```python
from build123d import *

# Parameters (mm, degrees)
SKETCH1_R           = 127.525
SKETCH1_R_2         = 124.525
BOSS_EXTRUDE1_DEPTH = 3
SKETCH2_R           = 1.5
BOSS_EXTRUDE2_DEPTH = 3
BOSS_EXTRUDE3_DEPTH = 3
FILLET1_R           = 5


with BuildPart() as part:
    # Sketch1 → Boss-Extrude1 (new body)
    with BuildSketch(Plane.XY):
        Circle(SKETCH1_R)
        Circle(SKETCH1_R_2, mode=Mode.SUBTRACT)
    extrude(amount=BOSS_EXTRUDE1_DEPTH)

    # Sketch2 → Boss-Extrude2 (add)
    with BuildSketch(Plane.XY.offset(3)):
        with BuildLine():
            Line((-6.110237311, 124.375), (-5, 119.525))
            ThreePointArc((-5, 119.525), (0, 114.525), (5, 119.525))
            Line((5, 119.525), (6.110237311, 124.375))
            ThreePointArc((6.110237311, 124.375), (0, 124.525), (-6.110237311, 124.375))
        make_face()
        with Locations((0, 119.525)):
            Circle(SKETCH2_R, mode=Mode.SUBTRACT)
        with BuildLine():
            Line((-119.525, 5), (-124.375, 6.110237311))
            ThreePointArc((-124.375, 6.110237311), (-124.525, 0), (-124.375, -6.110237311))
            Line((-124.375, -6.110237311), (-119.525, -5))
            ThreePointArc((-119.525, -5), (-114.525, 0), (-119.525, 5))
        make_face()
        with Locations((-119.525, 0)):
            Circle(SKETCH2_R, mode=Mode.SUBTRACT)
        with BuildLine():
            Line((-5, -119.525), (-6.110237311, -124.375))
            ThreePointArc((-6.110237311, -124.375), (0, -124.525), (6.110237311, -124.375))
            Line((6.110237311, -124.375), (5, -119.525))
            ThreePointArc((5, -119.525), (0, -114.525), (-5, -119.525))
        make_face()
        with Locations((0, -119.525)):
            Circle(SKETCH2_R, mode=Mode.SUBTRACT)
        with BuildLine():
            ThreePointArc((124.525, 0), (124.487494352, 3.056039103), (124.375, 6.110237311))
            Line((124.375, 6.110237311), (119.525, 5))
            ThreePointArc((119.525, 5), (114.525, 0), (119.525, -5))
            Line((119.525, -5), (124.375, -6.110237311))
            ThreePointArc((124.375, -6.110237311), (124.487494352, -3.056039103), (124.525, 0))
        make_face()
        with Locations((119.525, 0)):
            Circle(SKETCH2_R, mode=Mode.SUBTRACT)
    extrude(amount=-BOSS_EXTRUDE2_DEPTH)

    # Sketch3 → Boss-Extrude3 (add)
    with BuildSketch(Plane.XY.offset(3)):
        with BuildLine():
            ThreePointArc((122.429089666, 22.750684136), (119.019917661, 36.616046004), (114.045936469, 50))
            Line((114.045936469, 50), (114.045936469, -50))
            ThreePointArc((114.045936469, -50), (119.019917661, -36.616046004), (122.429089666, -22.750684136))
            ThreePointArc((122.429089666, -22.750684136), (115.850579192, -21.580706086), (119.525, -16))
            Line((119.525, -16), (119.525, -5))
            ThreePointArc((119.525, -5), (114.525, 0), (119.525, 5))
            Line((119.525, 5), (119.525, 16))
            ThreePointArc((119.525, 16), (115.850579192, 21.580706086), (122.429089666, 22.750684136))
        make_face()
        with BuildLine():
            ThreePointArc((123.166362087, 18.34455983), (121.690437522, 16.636834774), (119.525, 16))
            Line((119.525, 16), (119.525, 5))
            Line((119.525, 5), (124.375, 6.110237311))
            ThreePointArc((124.375, 6.110237311), (123.921754135, 12.242323195), (123.166362087, 18.34455983))
        make_face()
        with BuildLine():
            Line((119.525, -5), (119.525, -16))
            ThreePointArc((119.525, -16), (121.690437522, -16.636834774), (123.166362087, -18.34455983))
            ThreePointArc((123.166362087, -18.34455983), (123.921754135, -12.242323195), (124.375, -6.110237311))
            Line((124.375, -6.110237311), (119.525, -5))
        make_face()
    extrude(amount=-BOSS_EXTRUDE3_DEPTH)

    # Fillet1
    fillet1_edges = [part.edges().sort_by_distance(p)[0] for p in [
        (114.045936469, 50, 1.5),
        (114.045936469, -50, 1.5),
    ]]
    fillet(fillet1_edges, radius=FILLET1_R)


solid = part.part
```
The listing builds one solid part. Answer for the finished solid, in the listing's coordinates (mm). A direction names the side the tool comes from. Coordinates: 2 decimals unless noted, no trailing zeros. Loops run counter-clockwise (first coordinate to the right, second up) from the corner with the lowest first, then second, coordinate; pieces in that order, holes last. Notation, with made-up numbers: (19.5, -39.5) - (75.5, -39.5) arc R12 ccw to (75.5, -29.5) - close; hole circle Ø5 at (11, -39). An arc over 180 degrees is marked (long way). Use a Markdown table: item, result. Add a question column.
1) For faces 1 (the flat face through (122, 1, 3)), 2 (the cylindrical face through (69.42, -103.38, 1.48)), determine the directions among +Z, -Z, +X, -X, +Y, -Y from which every point of the face is accessible in a straight line to the end or side of a thin tool.
2) The part is cut by section C-C, the plane z = 1.35. Give the vertices of the cut face in (x, y) (3 decimals).
3) The part is cut by section B-B, the plane y = -70.5. Give the vertices of the cut face in (x, z), and give its area (3 significant figures).
4) The part is cut by section A-A, the plane x = -47. Give the vertices of the cut face in (y, z), and give its area (3 significant figures).
5) Find the intervals of material crossed by line 1 (Y direction, x = 0, z = 0.75) (3 decimals); line 2 (X direction, y = -63.5, z = 0.6); line 3 (Y direction, x = -90, z = 2.4), in increasing order.
6) The mould has two halves that part along X. Classify faces 3 (the flat face through (122, 1, 0)), 4 (the cylindrical face through (-27.645, -124.493, 1.479)), 5 (the cylindrical face through (-88.955, -87.14, 1.479)), 6 (the cylindrical face through (-87.14, 88.955, 1.479)): released by +X, released by -X, zero draft, split by the parting line, or undercut.
7) Given pin 1 (10.5 mm diameter, centred on x = 119.525, y = -20, fed in from -Z); pin 2 (1.5 mm diameter, centred on y = 40, z = 1, fed in from -X); pin 3 (1.8 mm diameter, centred on x = 119.525, y = 0, fed in from +Z); pin 4 (1.5 mm diameter, centred on x = -6, z = 1.5, fed in from +Y), each flat-ended and moving along its own axis, determine where each tip first touches the part or whether it passes through.
Here are the results:
| question | item | result |
|---|---|---|
| 1 | face 1 | +Z, +X, -X, +Y, -Y |
| 1 | face 2 | +Z, -Z |
| 2 | outline | circle Ø255.05 at (0, 0); hole (-124.375, -6.11) arc R124.525 ccw to (-6.11, -124.375) - (-5, -119.525) arc R5 cw to (5, -119.525) - (6.11, -124.375) arc R124.525 ccw to (113.608, -50.988) arc R5 ccw to (114.046, -48.941) - (114.046, 48.941) arc R5 ccw to (113.608, 50.988) arc R124.525 ccw to (6.11, 124.375) - (5, 119.525) arc R5 cw to (-5, 119.525) - (-6.11, 124.375) arc R124.525 ccw to (-124.375, 6.11) - (-119.525, 5) arc R5 cw to (-119.525, -5) - close; hole circle Ø3 at (-119.525, 0); hole circle Ø3 at (0, -119.525); hole circle Ø3 at (0, 119.525); hole circle Ø3 at (119.525, 0); hole (122.429, -22.751) arc R124.525 ccw to (123.166, -18.345) arc R4 ccw (long way) to start; hole (122.429, 22.751) arc R4 ccw (long way) to (123.166, 18.345) arc R124.525 ccw to start |
| 3 | outline | (-106.27, 0) - (-102.65, 0) - (-102.65, 3) - (-106.27, 3) - close; (102.65, 0) - (106.27, 0) - (106.27, 3) - (102.65, 3) - close |
| 3 | area | 21.7 mm^2 |
| 4 | outline | (-118.55, 0) - (-115.31, 0) - (-115.31, 3) - (-118.55, 3) - close; (115.31, 0) - (118.55, 0) - (118.55, 3) - (115.31, 3) - close |
| 4 | area | 19.4 mm^2 |
| 5 | line 1 | y = -127.525 to -121.025, -118.025 to -114.525, 114.525 to 118.025, 121.025 to 127.525 |
| 5 | line 2 | x = -110.59 to -107.12, 107.12 to 110.59 |
| 5 | line 3 | y = -90.35 to -86.06, 86.06 to 90.35 |
| 6 | face 3 | zero draft |
| 6 | face 4 | split by the parting line |
| 6 | face 5 | undercut |
| 6 | face 6 | undercut |
| 7 | pin 1 | stops at z = 0 |
| 7 | pin 2 | stops at x = -121.33 |
| 7 | pin 3 | passes through |
| 7 | pin 4 | stops at y = 127.42 |
